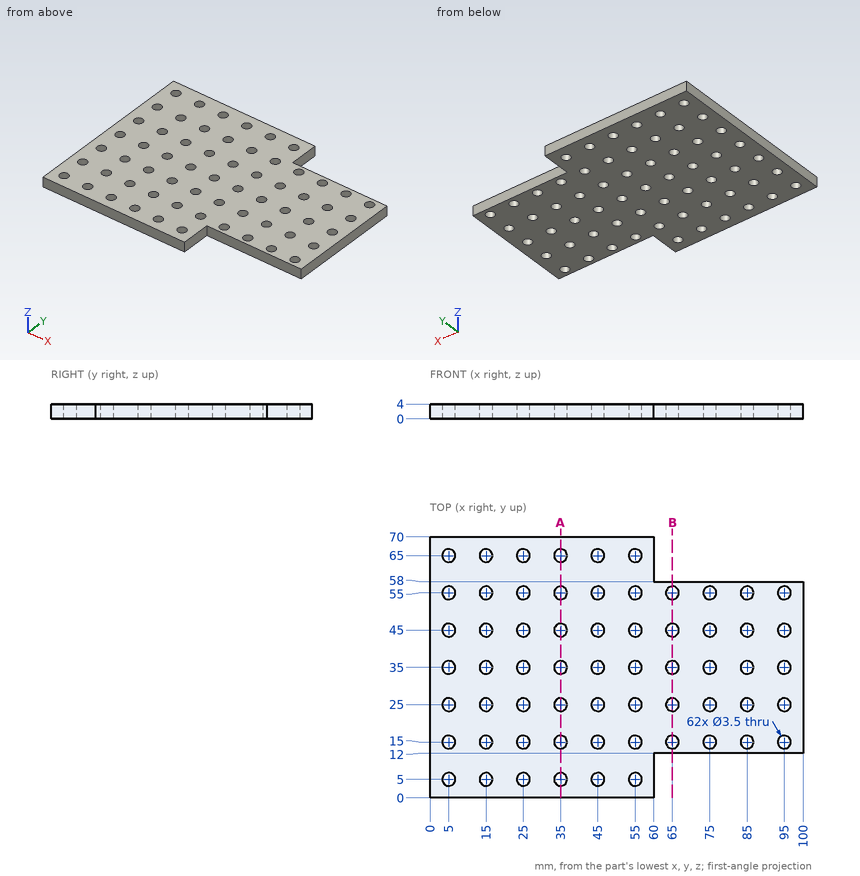
Part print with two shaded views. Sizes in mm from the minimum x, y, z corner. Coordinates: 2 decimals unless noted, no trailing zeros. Write each loop counter-clockwise with the first axis right and the second up, starting at its lowest first coordinate (ties: lowest second). Pieces come first, ordered by that corner, then holes. Notation, with made-up numbers: (57.5, 27) - (106.5, 27) arc R12 cw to (106.5, 37) - close; hole circle Ø11 at (35, -30). An arc over 180 degrees is marked (long way). One line per item, written item: value. Start each with the question number.
1. Slice it at B-B (x = 65). Write the cut outline in (y, z), plus the area to 3 significant figures.
2. Flat gauge pins, fed straight in: pin 1 (5.5 mm diameter, centred on x = 25, y = 45, fed in from -Z); pin 2 (1.5 mm diameter, centred on y = 61, z = 1, fed in from +X). Where does each tip first touch, or does it go through?
3. Slice it at A-A (x = 35). Count the separate pieces of the cut face and the enclosed holes in it, plus the area to 3 significant figures.
4. Probe line 1 (Y direction, x = 65, z = 3); line 2 (X direction, y = 60, z = 2.9); line 3 (Y direction, x = 70.5, z = 1.6). List the from-to ranges inside material, lowest first. Write a range as from..to.
Answers below:
1. outline: (12, 0) - (13.25, 0) - (13.25, 4) - (12, 4) - close; (16.75, 0) - (23.25, 0) - (23.25, 4) - (16.75, 4) - close; (26.75, 0) - (33.25, 0) - (33.25, 4) - (26.75, 4) - close; (36.75, 0) - (43.25, 0) - (43.25, 4) - (36.75, 4) - close; (46.75, 0) - (53.25, 0) - (53.25, 4) - (46.75, 4) - close; (56.75, 0) - (58, 0) - (58, 4) - (56.75, 4) - close
1. area: 114 mm^2
2. pin 1: stops at z = 0
2. pin 2: stops at x = 60
3. separate pieces: 8
3. enclosed holes: 0
3. area: 182 mm^2
4. line 1: y = 12..13.25, 16.75..23.25, 26.75..33.25, 36.75..43.25, 46.75..53.25, 56.75..58
4. line 2: x = 0..60
4. line 3: y = 12..58
